Read the model definition and answer for the solid it produces. Units are mm, in the model's axes. Face numbers are marked on the shaded views. Coordinates: 2 decimals unless noted, no trailing zeros. Loops run counter-clockwise (first coordinate to the right, second up) from the corner with the lowest first, then second, coordinate; pieces in that order, holes last. Notation, with made-up numbers: M 24,-19.75 L 28,-19.75 A20 cw 28,-7.75 Z; hole C 15,14.25 d8. An arc over 180 degrees is marked long. One line per item, written item: value. Start each with the question number.
1. Flat-ended cylindrical pins translate along their axes: pin 1 (3 mm diameter, centred on x = 0, y = -38.05, fed in from -Z); pin 2 (1.5 mm diameter, centred on x = -24, y = 13, fed in from +Z). Find the tip coordinate at first contact, or state that the pin passes through.
2. The part is cut by section A-A (z = 1.75). State how many separate pieces and enclosed holes the cut face has, then the cut area to 3 significant figures.
3. The part is cut by section B-B (y = -9.5). Write down the section's boundary in (x, z) (3 decimals), then the cut area to 3 significant figures.
4. Consider probe 1 along Y at (x, z) = (0, 1.9); probe 2 along X at (y, z) = (-22.5, 1) (3 decimals); probe 3 along Y at (x, z) = (-31.5, 1). Determine where each line is inside the solid, lowest interval first.
5. Determine the mould class of the marked faces 1 and 2 for opening direction Y: +Y half, -Y half, draft (parallel to the pull), parting line (faces both ways), or undercut.
6. The part is cut by section D-D (z = 8.25). Write down the section's boundary in (x, y) (3 decimals), then the cut area to 3 significant figures.
7. The part is cut by section C-C (x = 11). Write down the section's boundary in (y, z), then the cut area to 3 significant figures.
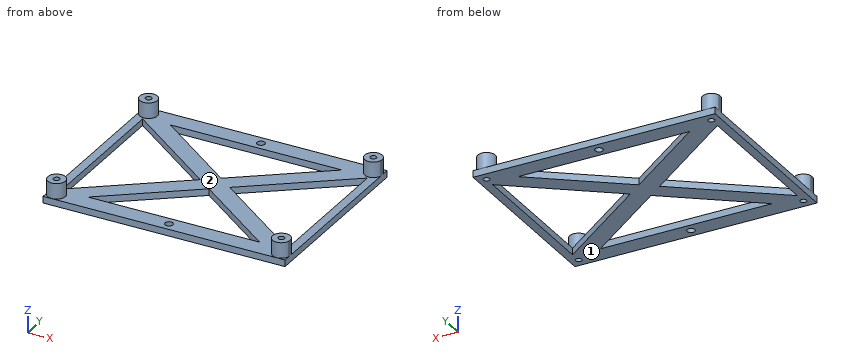
Autodesk Fusion 360 part; units mm, degrees
sketch "Sketch1" plane through (0, 0, 0) normal (0, 0, 1) x (1, 0, 0)
  line L0 (50.925, -38.05) -> (-50.925, -38.05) construction
  line L1 (-50.925, -38.05) -> (-50.925, 38.05) construction
  line L2 (-50.925, 38.05) -> (50.925, 38.05) construction
  line L3 (50.925, 38.05) -> (50.925, -38.05) construction
  line L4 (50.925, -38.05) -> (-50.925, 38.05) construction
  line L5 (-50.925, -38.05) -> (50.925, 38.05) construction
  circle A0 centre (-50.925, 38.05) radius 1.4
  circle A1 centre (50.925, 38.05) radius 1.4
  circle A2 centre (-50.925, -38.05) radius 1.4
  circle A3 centre (50.925, -38.05) radius 1.4
  line L6 (54.835, -42.15) -> (-54.835, -42.15)
  line L7 (-54.835, -42.15) -> (-54.835, 42.15)
  line L8 (-54.835, 42.15) -> (54.835, 42.15)
  line L9 (54.835, 42.15) -> (54.835, -42.15)
  line L10 (54.835, -42.15) -> (-54.835, 42.15) construction
  line L11 (-54.835, -42.15) -> (54.835, 42.15) construction
  circle A4 centre (-50.925, 38.05) radius 4
  circle A5 centre (-50.925, -38.05) radius 4
  circle A6 centre (50.925, -38.05) radius 4
  circle A7 centre (50.925, 38.05) radius 4
  line L12 (-50.925, 34.05) -> (50.925, 34.05)
  line L13 (50.925, 34.05) -> (50.925, -34.05)
  line L14 (50.925, -34.05) -> (-50.925, -34.05)
  line L15 (-50.925, -34.05) -> (-50.925, 34.05)
  line L16 (-50.925, 34.05) -> (50.925, -34.05) construction
  line L17 (50.925, 34.05) -> (-50.925, -34.05) construction
  line L18 (53.3192, 34.8457) -> (-48.5308, -41.2543)
  line L19 (48.5308, 41.2543) -> (-53.3192, -34.8457)
  line L20 (53.3192, -34.8457) -> (-48.5308, 41.2543)
  line L21 (-53.6868, 35.1565) -> (48.5301, -41.2538)
  circle A8 centre (0, 38.05) radius 1.75
  circle A9 centre (0, -38.05) radius 1.75
  dimension "d1" = 76.1
  dimension "d2" = 101.85
  dimension "d3" = 2.8
  dimension "d4" = 2.8
  dimension "d5" = 2.8
  dimension "d6" = 2.8
  dimension "d7" = 109.67
  dimension "d8" = 84.3
  dimension "d9" = 8
  dimension "d10" = 8
  dimension "d11" = 8
  dimension "d12" = 8
  dimension "d17" = 3.5
  dimension "d18" = 3.5
extrude "Extrude1" add sketch "Sketch1" along normal blind 3 contours L6 L7 L9 A5 A6 L14 L18 L21 | L9 A6 | L7 A5 | L9 A6 A7 L13 L18 L20 | A6 L14 L21 | L7 A4 A5 L15 L19 L21 | A5 L14 L18 | L9 A7 | A6 L13 L20 | L13 L14 L18 L20 L21 | L7 A4 L21 | A5 L15 L19 | L14 L15 L18 L19 L21 | L7 L8 L9 A4 A7 L12 L19 L20 | A7 L13 L18 | L18 L19 L20 L21 | A4 L21 | A7 L12 L19 | L12 L13 L18 L19 L20 | L12 L15 L19 L20 L21 | A4 L12 L20 | A4 L15 L21 | A8 | A9 picked at (53.9983, -38.05) picked at (-53.9983, -38.05) picked at (53.9983, 38.05)
extrude "Extrude2" add sketch "Sketch1" along normal blind 10 contours L9 A6 | L7 A5 | L9 A7 | L7 A4 L21 | A4 L21 picked at (53.9983, -38.05) picked at (-53.9983, -38.05) picked at (53.9983, 38.05)
extrude "Extrude3" cut sketch "Sketch1" along normal blind 7 contours A8 | A9
Answer block:
1. pin 1: passes through
1. pin 2: stops at z = 3
2. separate pieces: 1
2. enclosed holes: 10
2. area: 4,010 mm2
3. outline: M -54.835,0 L -50.925,0 L -50.925,3 L -54.835,3 Z; M -19.397,0 L -6.032,0 L -6.032,3 L -19.397,3 Z; M 6.052,0 L 19.397,0 L 19.397,3 L 6.052,3 Z; M 50.925,0 L 54.835,0 L 54.835,3 L 50.925,3 Z
3. area: 104 mm2
4. probe 1: y = -42.15 to -39.8, -36.3 to -34.05, -4.99 to 4.99, 34.05 to 36.3, 39.8 to 42.15
4. probe 2: x = -54.835 to -50.925, -36.796 to -23.431, 23.442 to 36.796, 50.925 to 54.835
4. probe 3: y = -42.15 to -34.05, -28.53 to -18.54, 18.57 to 28.53, 34.05 to 42.15
5. face 1: draft
5. face 2: undercut
6. outline: M -54.835,-38.894 A4 ccw long -54.835,-37.206 Z; M -54.835,37.206 A4 ccw long -54.835,38.894 Z; M 54.835,-38.894 L 54.835,-37.206 A4 ccw long Z; M 54.835,37.206 L 54.835,38.894 A4 ccw long Z; hole C -50.925,-38.05 d2.8; hole C -50.925,38.05 d2.8; hole C 50.925,-38.05 d2.8; hole C 50.925,38.05 d2.8
6. area: 176 mm2
7. outline: M -42.15,0 L -34.05,0 L -34.05,3 L -42.15,3 Z; M -13.2,0 L -3.23,0 L -3.23,3 L -13.2,3 Z; M 3.23,0 L 13.21,0 L 13.21,3 L 3.23,3 Z; M 34.05,0 L 42.15,0 L 42.15,3 L 34.05,3 Z
7. area: 108 mm2
